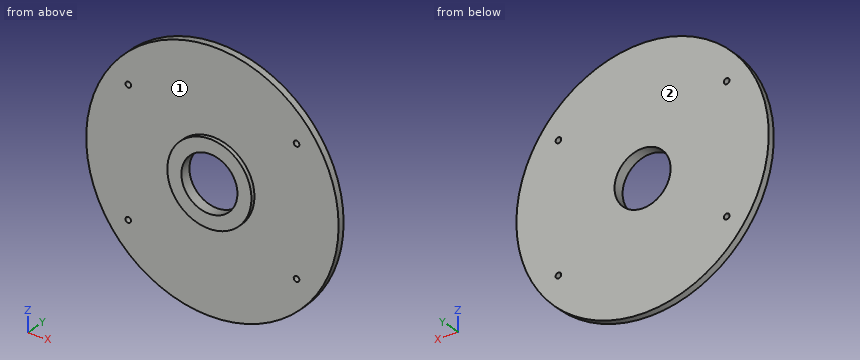
Solid Edge part; units mm, degrees
sketch "Sketch1" plane through (0, 0, 0) normal (0, -1, 0) x (1, 0, 0)
  circle A0 centre (60, 45) radius 2
  circle A1 centre (0, 0) radius 20
  circle A2 centre (0, 0) radius 90
  circle A3 centre (60, -45) radius 2
  circle A4 centre (-60, 45) radius 2
  circle A5 centre (-60, -45) radius 2
extrude "Protrusion1" add sketch "Sketch1" along normal blind 5
sketch "Sketch2" plane through (0, 0, 0) normal (0, -1, 0) x (1, 0, 0)
  circle A0 centre (0, 0) radius 30
  circle A1 centre (0, 0) radius 20
extrude "ExtrudedProtrusion_2" add sketch "Sketch2" along normal blind 8
Model file for the job. Use its own axes, mm. Face numbers are marked on the shaded views. A direction names the side the tool comes from. Give positions to 0.01 mm unless a question says otherwise; leave off trailing zeros. Loops run counter-clockwise (first coordinate to the right, second up) from the corner with the lowest first, then second, coordinate; pieces in that order, holes last.
1) Saw through at C-C (y = -2.25). Write the cut outline in (x, z), plus the area to 3 significant figures.
2) Flat gauge pins, fed straight in: pin 1 Ø6 at (x, z) = (31.5, -20.5) entering from -Y; pin 2 Ø6.5 at (x, z) = (-60, 45) entering from +Y; pin 3 Ø3 at (y, z) = (-1.5, -40.5) entering from -X; pin 4 Ø3 at (x, z) = (60, 45) entering from -Y. Where does each tip first touch, or does it go through?
3) Tool access for the marked faces 1 and 2: list every direction of +Z, -Z, +X, -X, +Y, -Y with a clear straight run to the whole face (end or side of a thin tool).
4) Saw through at B-B (x = 0). Write the cut outline in (y, z), plus the area to 3 significant figures.
5) Wall check: line 1 (Z direction, x = 60, y = -2.35); line 2 (Z direction, x = 0, y = -4.5); line 3 (Y direction, x = 5, z = -81.5). Give the ranges that are in metal, low to high.
6) Saw through at A-A (z = 0). Write the cut outline in (x, y).
7) Saw through at D-D (z = -22.5). Write the cut outline in (x, y), plus the area to 3 significant figures.
Answer block:
1. outline: circle Ø180 at (0, 0); hole circle Ø4 at (-60, -45); hole circle Ø4 at (-60, 45); hole circle Ø40 at (0, 0); hole circle Ø4 at (60, -45); hole circle Ø4 at (60, 45)
1. area: 24,100 mm2
2. pin 1: stops at y = -5
2. pin 2: stops at y = 0
2. pin 3: stops at x = -81.11
2. pin 4: passes through
3. face 1: -Y
3. face 2: +Z, -Z, +X, -X, +Y
4. outline: (-8, -30) - (-5, -30) - (-5, -90) - (0, -90) - (0, -20) - (-8, -20) - close; (-8, 20) - (0, 20) - (0, 90) - (-5, 90) - (-5, 30) - (-8, 30) - close
4. area: 760 mm2
5. line 1: z = -67.08 to -47, -43 to 43, 47 to 67.08
5. line 2: z = -90 to -20, 20 to 90
5. line 3: y = -5 to 0
6. outline: (-90, -5) - (-30, -5) - (-30, -8) - (-20, -8) - (-20, 0) - (-90, 0) - close; (20, -8) - (30, -8) - (30, -5) - (90, -5) - (90, 0) - (20, 0) - close
7. outline: (-87.14, -5) - (-19.84, -5) - (-19.84, -8) - (19.84, -8) - (19.84, -5) - (87.14, -5) - (87.14, 0) - (-87.14, 0) - close
7. area: 990 mm2
